Could you check a few things on this model? Use its own coordinates, in mm. Face numbers are marked on the shaded views. A direction names the side the tool comes from. Coordinates: 2 decimals unless noted, no trailing zeros. Write each loop counter-clockwise with the first axis right and the second up, starting at its lowest first coordinate (ties: lowest second). Pieces come first, ordered by that corner, then holes.
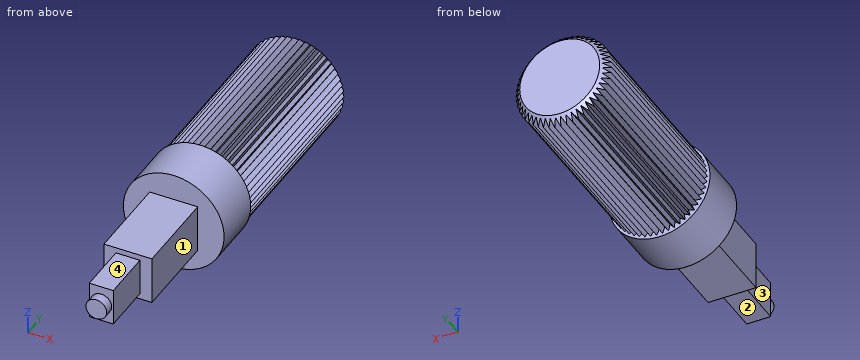
```python
from build123d import *

# Parameters (mm, degrees)
SKETCH_1_R               = 3.15
EXTRUDE_1_DEPTH          = 3.2
SKETCH_2_R               = 3
EXTRUDE_2_DEPTH          = 12
CHAMFER_1_SIZE           = 0.5
SKETCH_3_W               = 3
SKETCH_3_H               = 3
EXTRUDE_3_DEPTH          = 5.5
SKETCH_4_W               = 1.5
SKETCH_4_H               = 2.3
EXTRUDE_4_DEPTH          = 3.2
SKETCH_5_R               = 0.65
EXTRUDE_5_DEPTH          = 0.6
CUT_EXTRUDE_1_DEPTH      = 12
PATTERN_CIRCULAR_1_COUNT = 50


with BuildPart() as part:
    # Эскиз1 → Бобышка-Вытянуть1 (new body)
    with BuildSketch(Plane(origin=(0, 0, 0), x_dir=(1, 0, 0), z_dir=(0, 1, 0))):
        Circle(SKETCH_1_R)
    extrude(amount=EXTRUDE_1_DEPTH)

    # Эскиз2 → Бобышка-Вытянуть2 (add)
    with BuildSketch(Plane(origin=(0, 3.2, 0), x_dir=(1, 0, 0), z_dir=(0, 1, 0))):
        Circle(SKETCH_2_R)
    extrude(amount=EXTRUDE_2_DEPTH)

    # Фаска1
    chamfer_1_edges = [part.edges().sort_by_distance(p)[0] for p in [
        (-3, 15.2, 0),
    ]]
    chamfer(chamfer_1_edges, length=CHAMFER_1_SIZE)

    # Эскиз3 → Бобышка-Вытянуть3 (add)
    with BuildSketch(Plane.XZ):
        Rectangle(SKETCH_3_W, SKETCH_3_H)
    extrude(amount=EXTRUDE_3_DEPTH)

    # Эскиз4 → Бобышка-Вытянуть4 (add)
    with BuildSketch(Plane.XZ.offset(5.5)):
        Rectangle(SKETCH_4_W, SKETCH_4_H)
    extrude(amount=EXTRUDE_4_DEPTH)

    # Эскиз5 → Бобышка-Вытянуть5 (add)
    with BuildSketch(Plane.XZ.offset(8.7)):
        Circle(SKETCH_5_R)
    extrude(amount=EXTRUDE_5_DEPTH)

    # Эскиз7 → Вырез-Вытянуть1 (cut)
    with BuildSketch(Plane(origin=(0, 15.2, 0), x_dir=(1, 0, 0), z_dir=(0, 1, 0))):
        Polygon((0, 2.612170904), (-0.2, 3.012170904), (0.2, 3.012170904), align=None)
    cut_extrude_1 = extrude(amount=-CUT_EXTRUDE_1_DEPTH, mode=Mode.SUBTRACT)

    # Круговой массив1: Вырез-Вытянуть1 ×50 about axis
    pattern_circular_1_axis = Axis((0, 0, 0), (0, 1, 0))
    for i in range(1, PATTERN_CIRCULAR_1_COUNT):
        add(cut_extrude_1.rotate(pattern_circular_1_axis, i * 360 / PATTERN_CIRCULAR_1_COUNT), mode=Mode.SUBTRACT)


solid = part.part
```
Item 1: I want a section at A-A, the plane y = -6.25. List the corners of the cut face in (x, z) for me, then the cut area to 3 significant figures.
Item 2: Which directions (+Z, -Z, +X, -X, +Y, -Y) give clear straight access to the entire face, cutting with the end or side of a thin tool? Please do the marked faces 1, 2, 3 and 4.
Item 3: If I drill on line 1 along Y through (x, z) = (0.25, 2.25); line 2 along Y through (x, z) = (1.75, -2.5); line 3 along Z through (x, y) = (2, 1.25), over which ranges is the centre line in solid material (lowest first)?
Item 4: Will these pins go through, and if not, where does the flat tip stop? pin 1 Ø1.8 at (y, z) = (-8, -0.5) entering from +X; pin 2 Ø1.5 at (x, y) = (0, -4) entering from +Z; pin 3 Ø3.5 at (y, z) = (-4, 0) entering from -X.
Taken from the geometry:
1. outline: (-0.75, -1.15) - (0.75, -1.15) - (0.75, 1.15) - (-0.75, 1.15) - close
1. area: 3.45 mm2
2. face 1: +Z, -Z, +X, -Y
2. face 2: -Z, +X, -X, -Y
2. face 3: +Z, -Z, -X, -Y
2. face 4: +Z, +X, -X, -Y
3. line 1: y = 0 to 15.2
3. line 2: y = 0 to 3.2
3. line 3: z = -2.43 to 2.43
4. pin 1: stops at x = 0.75
4. pin 2: stops at z = 1.5
4. pin 3: stops at x = -1.5
